Here's how the part is built. I have some questions about the finished solid (model axes, mm). A direction names the side the tool comes from. Round coordinates to 2 decimals unless told otherwise and drop trailing zeros. Order: outer loops, then holes, each group sorted by start corner. A loop starts at its lowest first (then second) coordinate and runs counter-clockwise, first axis right, second up. Notation, with made-up numbers: M 69.5,32 L 107.5,32 A15 cw 107.5,45 Z; hole C 36.5,88.5 d1. An arc over 180 degrees is marked long. Write item = value, one per line. Start each with the question number.
Item 1: We'd pull the mould along X, two halves only. Please class faces 3 (the face through (7.08, 21.056, 7.606)), 4 (the face through (28, -25, 9)), 5 (the face through (32.73, -21.06, 15.38)): pulls with the +X half, pulls with the -X half, needs draft (parallel to the pull), parting line crosses it, or undercut.
Item 2: I'm going to push flat-ended pins straight in: P1, Ø6, axis at x = -13.5, y = 1, coming from the -Z side; P2, Ø1.5, axis at x = -6, z = -13, coming from the +Y side; P3, Ø3, axis at x = -12, z = 8.5, coming from the +Y side; P4, Ø10, axis at x = 32, y = -16.5, coming from the +Z side. Where does each tip first touch, or does it pass through?
Item 3: For faces 1 (the face through (28, 17, 9)), 2 (the face through (28, 25, 9)), which set-ups out of +Z, -Z, +X, -X, +Y, -Y let a thin tool reach every point of the face, with its end or its side?
Item 4: I want a section at A-A, the plane z = -3. List the corners of the cut face in (x, y) for me, plus the area to 3 significant figures.
Item 5: I want a section at D-D, the plane x = -5. List the corners of the cut face in (y, z) for me, plus the area to 3 significant figures.
Item 6: Please list where these lines run through material, in increasing order: L1, parallel to Z at x = 17, y = -19; L2, parallel to Y at x = 4.5, z = 15.5; L3, parallel to X at y = -22.25, z = 0.
Item 7: I want a section at B-B, the plane x = 10.5. List the corners of the cut face in (y, z) for me, plus the area to 3 significant figures.
Autodesk Inventor part; units mm, degrees
ref_plane "YZ Plane" through (0, 0, 0) normal (1, 0, 0) x (0, 1, 0)
ref_plane "XZ Plane" through (0, 0, 0) normal (0, 1, 0) x (-1, 0, 0)
ref_plane "XY Plane" through (0, 0, 0) normal (0, 0, 1) x (1, 0, 0)
sketch "草圖1" plane through (0, 0, 0) normal (0, 0, 1) x (1, 0, 0)
  arc A0 (0, 17) -> (0, -17) centre (0, 0) ccw
  arc A1 (0, 25) -> (0, -25) centre (0, 0) ccw
  line L0 (0, 27.0608) -> (0, -29.1984) construction
  line L1 (0, 25) -> (28, 25)
  line L2 (0, 17) -> (28, 17)
  line L3 (28, 25) -> (39, 25)
  line L4 (28, 17) -> (39, 17)
  line L5 (39, 17) -> (39, 25)
  line L6 (0, 0) -> (33.5, 0) construction
  line L7 (0, -25) -> (28, -25)
  line L8 (0, -17) -> (28, -17)
  line L9 (28, -25) -> (39, -25)
  line L10 (28, -17) -> (39, -17)
  line L11 (39, -17) -> (39, -25)
  dimension "d0" = 34
  dimension "d1" = 50
  dimension "d2" = 28
  dimension "d3" = 11
  dimension "d4" = 11
  dimension "d5" = 34
extrude "擠出1" add sketch "草圖1" along normal mid plane 44
fillet "圓角1" radius 22 4 edges at (39, 21, 22) (39, 21, -22) (39, -21, 22) (39, -21, -22)
sketch "草圖2" plane through (0, 25, 22) normal (0, 1, 0) x (1, 0, 0)
  arc A0 (17, 0) -> (17, 44) centre (17, 22) ccw
  circle A1 centre (17, 22) radius 12.5
  point P0 (0, 22)
  dimension "d9" = 25
extrude "擠出2" cut sketch "草圖2" against normal blind 60
properties part number "410571040練習三"
Filled in:
q1.face_3 = undercut
q1.face_4 = needs draft
q1.face_5 = pulls with the +X half
q2.P1 = through
q2.P2 = 24.44
q2.P3 = 22.69
q2.P4 = 19.58
q3.face_1 = +Z, -Z, +X
q3.face_2 = +Z, -Z, +X, -X, +Y
q4.outline = M 0,-25 L 4.87,-25 L 4.87,-17 L 0,-17 A17 cw 0,17 L 4.87,17 L 4.87,25 L 0,25 A25 ccw Z; M 29.13,-25 L 38.79,-25 L 38.79,-17 L 29.13,-17 Z; M 29.13,17 L 38.79,17 L 38.79,25 L 29.13,25 Z
q4.area = 760 mm^2
q5.outline = M -24.49,-22 L -16.25,-22 L -16.25,22 L -24.49,22 Z; M 16.25,-22 L 24.49,-22 L 24.49,22 L 16.25,22 Z
q5.area = 726 mm^2
q6.L1 = -22 to -12.5, 12.5 to 22
q6.L2 = -25 to -17, 17 to 25
q6.L3 = -11.4 to 4.5, 29.5 to 39
q7.outline = M -25,-22 L -17,-22 L -17,-10.68 L -25,-10.68 Z; M -25,10.68 L -17,10.68 L -17,22 L -25,22 Z; M 17,-22 L 25,-22 L 25,-10.68 L 17,-10.68 Z; M 17,10.68 L 25,10.68 L 25,22 L 17,22 Z
q7.area = 362 mm^2
